```python
from build123d import *

# Parameters (mm, degrees)
SKETCH1_R           = 9.75
BOSS_EXTRUDE1_DEPTH = 1
CUT_EXTRUDE1_DEPTH  = 3


with BuildPart() as part:
    # Sketch1 → Boss-Extrude1 (new body)
    with BuildSketch(Plane(origin=(0, 0, 0), x_dir=(1, 0, 0), z_dir=(0, 1, 0))):
        with Locations(Location((0, 0, 0), (0, 0, 270))):
            Circle(SKETCH1_R)
    extrude(amount=BOSS_EXTRUDE1_DEPTH)

    # Sketch2 → Cut-Extrude1 (cut)
    with BuildSketch(Plane(origin=(0, 1, 0), x_dir=(1, 0, 0), z_dir=(0, 1, 0))):
        with BuildLine():
            Line((-2.19089023, 0.2), (0, 0.2))
            Line((0, 0.2), (2.19089023, 0.2))
            ThreePointArc((2.19089023, 0.2), (0, 2.2), (-2.19089023, 0.2))
        make_face()
        with BuildLine():
            Line((2.19089023, -0.2), (-2.19089023, -0.2))
            ThreePointArc((-2.19089023, -0.2), (0, -2.2), (2.19089023, -0.2))
        make_face()
    extrude(amount=-CUT_EXTRUDE1_DEPTH, mode=Mode.SUBTRACT)


solid = part.part
```
Could you check a few things on this model? Use its own coordinates, in mm. A direction names the side the tool comes from. Coordinates: 2 decimals unless noted, no trailing zeros. Write each loop counter-clockwise with the first axis right and the second up, starting at its lowest first coordinate (ties: lowest second). Pieces come first, ordered by that corner, then holes. Notation, with made-up numbers: M 44,-6 L 94,-6 A19 cw 94,9 Z; hole C 42,16.5 d7. An arc over 180 degrees is marked long. Answer as CSV lines item,"result". Start each with the question number.
1) I want a section at A-A, the plane x = 0. Please give me the cut outline in (y, z).
2) We'd pull the mould along Z, two halves only. Please class faces 1 (the cylindrical face through (9.667, 0.493, -1.269)), 2 (the flat face through (0, 0.5, -0.2)), 3 (the flat face through (0, 0, 0)): +Z half, -Z half, draft (parallel to the pull), parting line (faces both ways), or undercut.
3) For faces 4 (the flat face through (0, 0.5, 0.2)), 5 (the flat face through (0, 1, 0)), which set-ups out of +Z, -Z, +X, -X, +Y, -Y let a thin tool reach every point of the face, with its end or its side?
4) I want a section at C-C, the plane x = 3. Please give me the cut outline in (y, z).
5) I want a section at D-D, the plane x = 6. Please give me the cut outline in (y, z), and give its area (3 significant figures).
6) I want a section at B-B, the plane y = 0.3. Please give me the cut outline in (x, z), and give its area (3 significant figures).
7) Please list where these lines run through material, in increasing order: line 1 (X direction, y = 0.45, z = 0.75); line 2 (Z direction, x = 7.5, y = 0.25); line 3 (X direction, y = 0.8, z = -4.25). Write a range as from..to.
8) For P1, Ø10, axis at x = -2, z = -5, coming from the -Y side, with a flat end and sliding along its axis, tell me the tip position at first contact or that it passes through.
Data:
1,outline,"M 0,-9.75 L 1,-9.75 L 1,-2.2 L 0,-2.2 Z; M 0,-0.2 L 1,-0.2 L 1,0.2 L 0,0.2 Z; M 0,2.2 L 1,2.2 L 1,9.75 L 0,9.75 Z"
2,face 1,"parting line"
2,face 2,"undercut"
2,face 3,"draft"
3,face 4,"+Y, -Y"
3,face 5,"+Z, -Z, +X, -X, +Y"
4,outline,"M 0,-9.28 L 1,-9.28 L 1,9.28 L 0,9.28 Z"
5,outline,"M 0,-7.69 L 1,-7.69 L 1,7.69 L 0,7.69 Z"
5,area,"15.4 mm^2"
6,outline,"C 0,0 d19.5; hole M -2.19,-0.2 A2.2 ccw 2.19,-0.2 Z; hole M -2.19,0.2 L 2.19,0.2 A2.2 ccw Z"
6,area,"285 mm^2"
7,line 1,"x = -9.72..-2.07, 2.07..9.72"
7,line 2,"z = -6.23..6.23"
7,line 3,"x = -8.77..8.77"
8,P1,"stops at y = 0"
